Check sheet for the drawn part. Datum: minimum x, y, z corner. Units: mm. Give positions to 0.01 mm unless a question says otherwise; leave off trailing zeros. Loops run counter-clockwise (first coordinate to the right, second up) from the corner with the lowest first, then second, coordinate; pieces in that order, holes last.
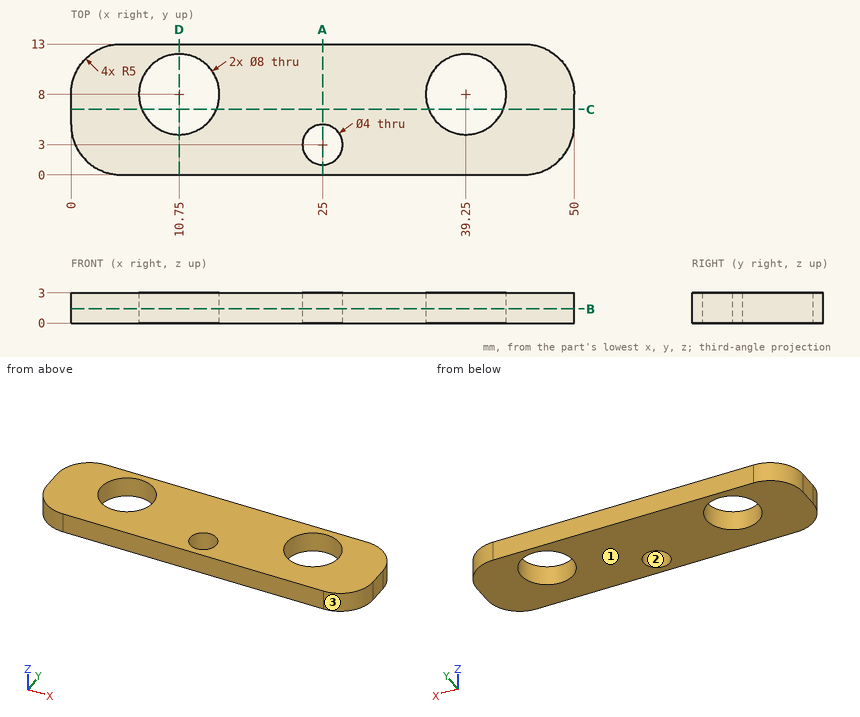
(1) Section check C-C on y = 6.5. Record the boundary of the cut face in (x, z).
(2) Release check for a two-part mould opening along Y. For the marked faces 1, 2 and 3 record: pulls with the +Y half, pulls with the -Y half, needs draft (parallel to the pull), parting line crosses it, or undercut.
(3) Section check D-D on x = 10.75. Record the boundary of the cut face in (y, z), plus the area to 3 significant figures.
(4) Material ranges on line 1 (X direction, y = 6.5, z = 0.55); line 2 (Y direction, x = 10.75, z = 1.9); line 3 (Y direction, x = 25, z = 1.05), recorded low to high.
(5) Section check A-A on x = 25. Record the boundary of the cut face in (y, z).
(6) Gauge pin test, flat end, axial feed: pin 1 Ø6.5 at (x, y) = (10.75, 8) entering from +Z. Record the tip position at first contact, or that the pin passes through.
(7) Section check B-B on z = 1.4. Record the boundary of the cut face in (x, y), plus the area to 3 significant figures.
Computed values:
1. outline: (0, 0) - (7.04, 0) - (7.04, 3) - (0, 3) - close; (14.46, 0) - (35.54, 0) - (35.54, 3) - (14.46, 3) - close; (42.96, 0) - (50, 0) - (50, 3) - (42.96, 3) - close
2. face 1: needs draft
2. face 2: undercut
2. face 3: pulls with the -Y half
3. outline: (0, 0) - (4, 0) - (4, 3) - (0, 3) - close; (12, 0) - (13, 0) - (13, 3) - (12, 3) - close
3. area: 15.0 mm2
4. line 1: x = 0 to 7.04, 14.46 to 35.54, 42.96 to 50
4. line 2: y = 0 to 4, 12 to 13
4. line 3: y = 0 to 1, 5 to 13
5. outline: (0, 0) - (1, 0) - (1, 3) - (0, 3) - close; (5, 0) - (13, 0) - (13, 3) - (5, 3) - close
6. pin 1: passes through
7. outline: (0, 5) arc R5 ccw to (5, 0) - (45, 0) arc R5 ccw to (50, 5) - (50, 8) arc R5 ccw to (45, 13) - (5, 13) arc R5 ccw to (0, 8) - close; hole circle Ø8 at (10.75, 8); hole circle Ø4 at (25, 3); hole circle Ø8 at (39.25, 8)
7. area: 515 mm2
